from build123d import *

# Parameters (mm, degrees)
CROQUIS1_W              = 20
CROQUIS1_H              = 10
CROQUIS1_R              = 1.25
SALIENTE_EXTRUIR1_DEPTH = 2
CROQUIS2_W              = 2
CROQUIS2_H              = 10
SALIENTE_EXTRUIR2_DEPTH = 11
CROQUIS3_W              = 20
CROQUIS3_H              = 10
CROQUIS3_R              = 1.25
SALIENTE_EXTRUIR3_DEPTH = 2
CROQUIS4_W              = 2
CROQUIS4_H              = 11
SALIENTE_EXTRUIR4_DEPTH = 17
CROQUIS5_W              = 11
CROQUIS5_H              = 2
SALIENTE_EXTRUIR5_DEPTH = 6
CROQUIS6_W              = 11
CROQUIS6_H              = 2
SALIENTE_EXTRUIR6_DEPTH = 6
CROQUIS7_W              = 24
CROQUIS7_H              = 11
CROQUIS7_W_2            = 20
CROQUIS7_H_2            = 7
CORTAR_EXTRUIR1_DEPTH   = 1
CROQUIS8_R              = 1.5
CORTAR_EXTRUIR2_DEPTH   = 11
CHAFL_N1_SIZE           = 0.5


with BuildPart() as part:
    # Croquis1 → Saliente-Extruir1 (new body)
    with BuildSketch(Plane.XY):
        with Locations((10, 5)):
            Rectangle(CROQUIS1_W, CROQUIS1_H)
        with Locations((5.25, 2.3)):
            Circle(CROQUIS1_R, mode=Mode.SUBTRACT)
        with Locations((14.75, 2.3)):
            Circle(CROQUIS1_R, mode=Mode.SUBTRACT)
    extrude(amount=SALIENTE_EXTRUIR1_DEPTH)

    # Croquis2 → Saliente-Extruir2 (add)
    with BuildSketch(Plane.XY.offset(2)):
        with Locations((-1, 5)):
            Rectangle(CROQUIS2_W, CROQUIS2_H)
        with Locations((21, 5)):
            Rectangle(CROQUIS2_W, CROQUIS2_H)
    extrude(amount=-SALIENTE_EXTRUIR2_DEPTH)



with BuildPart() as body_2:
    # Croquis3 → Saliente-Extruir3 (new body)
    with BuildSketch(Plane(origin=(0, 0, -9), x_dir=(-1, 0, 0), z_dir=(0, 0, -1))):
        with Locations((-10, 5)):
            Rectangle(CROQUIS3_W, CROQUIS3_H)
        with Locations(Location((-5.25, 2.3, 0), (0, 0, 180))):
            Circle(CROQUIS3_R, mode=Mode.SUBTRACT)
        with Locations(Location((-14.75, 2.3, 0), (0, 0, 180))):
            Circle(CROQUIS3_R, mode=Mode.SUBTRACT)
    extrude(amount=-SALIENTE_EXTRUIR3_DEPTH)


with BuildPart() as part_1:
    add(part.part)

    add(body_2.part)  # Saliente-Extruir4 merges body 2
    # Croquis4 → Saliente-Extruir4 (add)
    with BuildSketch(Plane.XZ):
        with Locations((-1, -3.5)):
            Rectangle(CROQUIS4_W, CROQUIS4_H)
        with Locations((21, -3.5)):
            Rectangle(CROQUIS4_W, CROQUIS4_H)
    extrude(amount=SALIENTE_EXTRUIR4_DEPTH)

    # Croquis5 → Saliente-Extruir5 (add)
    with BuildSketch(Plane(origin=(22, 0, 0), x_dir=(0, 0, -1), z_dir=(1, 0, 0))):
        with Locations((3.5, -16)):
            Rectangle(CROQUIS5_W, CROQUIS5_H)
    extrude(amount=SALIENTE_EXTRUIR5_DEPTH)

    # Croquis6 → Saliente-Extruir6 (add)
    with BuildSketch(Plane.ZY.offset(2)):
        with Locations((-3.5, -16)):
            Rectangle(CROQUIS6_W, CROQUIS6_H)
    extrude(amount=SALIENTE_EXTRUIR6_DEPTH)

    # Croquis7 → Cortar-Extruir1 (cut)
    with BuildSketch(Plane(origin=(0, 10, 0), x_dir=(1, 0, 0), z_dir=(0, 1, 0))):
        with Locations((10, 3.5)):
            Rectangle(CROQUIS7_W, CROQUIS7_H)
        with Locations((10, 3.5)):
            Rectangle(CROQUIS7_W_2, CROQUIS7_H_2, mode=Mode.SUBTRACT)
    extrude(amount=-CORTAR_EXTRUIR1_DEPTH, mode=Mode.SUBTRACT)

    # Croquis8 → Cortar-Extruir2 (cut)
    with BuildSketch(Plane(origin=(0, -15, 0), x_dir=(1, 0, 0), z_dir=(0, 1, 0))):
        with Locations(Location((-5, 3.5, 0), (0, 0, 180))):
            Circle(CROQUIS8_R)
        with Locations(Location((25, 3.5, 0), (0, 0, 180))):
            Circle(CROQUIS8_R)
    extrude(amount=-CORTAR_EXTRUIR2_DEPTH, mode=Mode.SUBTRACT)

    # Chaflán1
    chafl_n1_edges = [part_1.edges().sort_by_distance(p)[0] for p in [
        (-2, -15, -3.5),
        (0, 0, 1),
        (0, 0, -8),
        (20, 0, 1),
        (20, 0, -8),
        (22, -15, -3.5),
    ]]
    chamfer(chafl_n1_edges, length=CHAFL_N1_SIZE)


solid = part_1.part
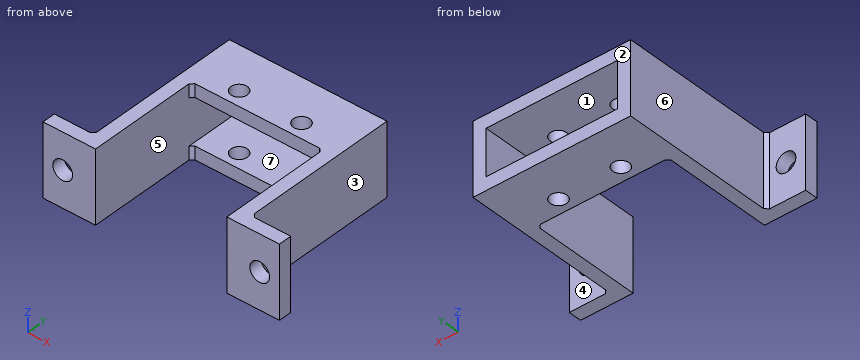
Build history of the part. All positions in model axes, mm. Face numbers are marked on the shaded views. A direction names the side the tool comes from. Coordinates: 2 decimals unless noted, no trailing zeros. Order: outer loops, then holes, each group sorted by start corner. A loop starts at its lowest first (then second) coordinate and runs counter-clockwise, first axis right, second up. Notation, with made-up numbers: M 55,-2 L 59,-2 A20 cw 59,34 Z; hole C 56.25,40.5 d10. An arc over 180 degrees is marked long. One line per question, with ' | ' between items. Start each with the question number.
Q1. Saw through at A-A (x = 12). List the corners of the cut face in (y, z), then the cut area to 3 significant figures.
Q2. Saw through at B-B (z = -7.5). List the corners of the cut face in (x, y).
Q3. Saw through at D-D (y = 2.3). List the corners of the cut face in (x, z).
Q4. 3-axis set-ups, long thin cutter, end or side, ignore diameter. For the marked faces 4, 5, 6 and 7: which of +Z, -Z, +X, -X, +Y, -Y reach the whole face in a straight line?
Q5. Probe L1, parallel to X at y = 0.5, z = -1.75; L2, parallel to Y at x = 26.5, z = 1.25; L3, parallel to Z at x = -5, y = -15.85. List the from-to ranges inside material, lowest first. Write a range as from..to.
Q6. Flat gauge pins, fed straight in: pin 1 Ø5.5 at (y, z) = (-2.5, -3) entering from -X; pin 2 Ø5.5 at (y, z) = (-3, -4.5) entering from +X; pin 3 Ø3 at (x, y) = (5.25, 2.3) entering from -Z; pin 4 Ø1 at (x, z) = (11, -8.5) entering from -Y. Where does each tip first touch, or does it go through?
Q7. Two-plate mould, pull along X, no slides. Class the marked faces 1, 2 and 3: +X half, -X half, draft (parallel to the pull), parting line (faces both ways), or undercut.
Q8. Saw through at C-C (x = 5.25). List the corners of the cut face in (y, z).
Check values:
1) outline: M 0,-9 L 9,-9 L 9,-7 L 0,-7 Z; M 0,0 L 9,0 L 9,2 L 0,2 Z | area: 36.0 mm2
2) outline: M -8,-17 L 0,-17 L 0,-0.5 L 0.5,0 L 19.5,0 L 20,-0.5 L 20,-17 L 28,-17 L 28,-15 L 22.5,-15 L 22,-14.5 L 22,9 L -2,9 L -2,-14.5 L -2.5,-15 L -8,-15 Z; hole C 5.25,2.3 d2.5; hole C 14.75,2.3 d2.5
3) outline: M -2,-9 L 4,-9 L 4,-7 L 0,-7 L 0,0 L 4,0 L 4,2 L -2,2 Z; M 6.5,-9 L 13.5,-9 L 13.5,-7 L 6.5,-7 Z; M 6.5,0 L 13.5,0 L 13.5,2 L 6.5,2 Z; M 16,-9 L 22,-9 L 22,2 L 16,2 L 16,0 L 20,0 L 20,-7 L 16,-7 Z
4) face 4: +Z, -Z, +X, +Y | face 5: -Y | face 6: +Z, -Z, -X, +Y | face 7: +Y, -Y
5) L1: x = -2..0, 20..22 | L2: y = -17..-15 | L3: z = -9..-5, -2..2
6) pin 1: stops at x = -2 | pin 2: stops at x = 22 | pin 3: stops at z = -9 | pin 4: stops at y = 0
7) face 1: undercut | face 2: draft | face 3: +X half
8) outline: M 0,-9 L 1.05,-9 L 1.05,-7 L 0,-7 Z; M 0,0 L 1.05,0 L 1.05,2 L 0,2 Z; M 3.55,-9 L 9,-9 L 9,-7 L 3.55,-7 Z; M 3.55,0 L 9,0 L 9,2 L 3.55,2 Z
